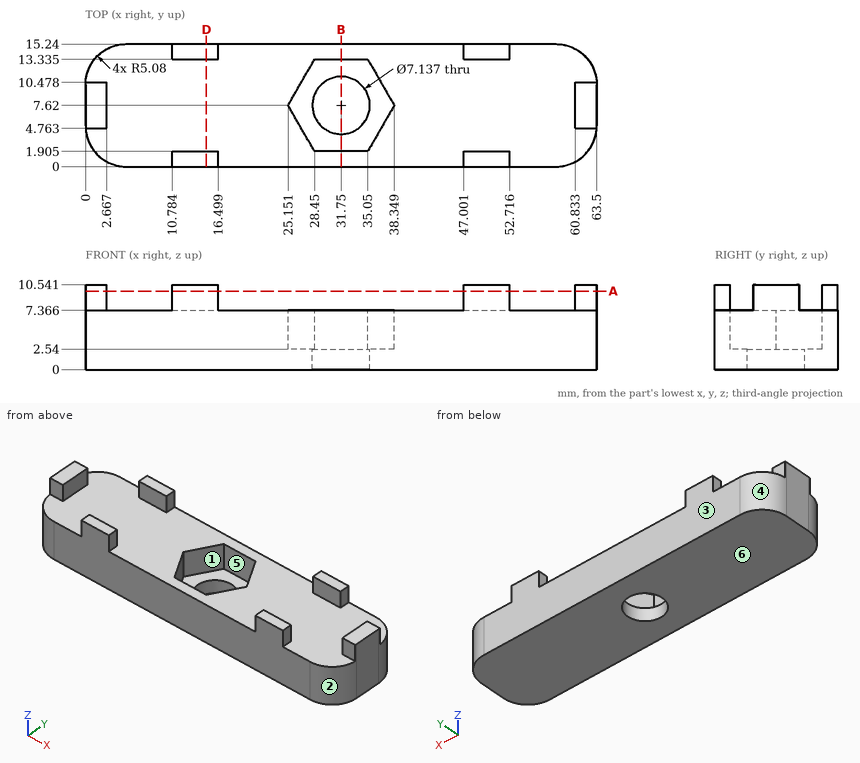
Verification items for this drawing (mm, ordinates from the low corner). A direction names the side the tool comes from. Coordinates: 2 decimals unless noted, no trailing zeros. Write each loop counter-clockwise with the first axis right and the second up, starting at its lowest first coordinate (ties: lowest second). Pieces come first, ordered by that corner, then holes. Notation, with made-up numbers: M 18.25,46.5 L 51.25,46.5 A22 cw 51.25,54.5 Z; hole C 36,4 d7. An arc over 180 degrees is marked long. Answer as a JSON object with one key per item and string values. Group by question number.
(1) Tool access check on the marked faces 5 and 6. Record the directions out of +Z, -Z, +X, -X, +Y, -Y that give a thin tool (end or side, any length) a straight path to the whole face; none if there is none.
(2) Cross-section at B-B, the plane x = 31.75. Record the cut outline in (y, z) (1 decimal).
(3) Gauge pin test, flat ends, axial feed: pin 1 (3 mm diameter, centred on x = 0.5, z = 9.5, fed in from -Y); pin 2 (0.6 mm diameter, centred on y = 14, z = 9, fed in from -X); pin 3 (1 mm diameter, centred on x = 51.5, y = 3, fed in from +Z). Record the tip position at first contact, or that the pin passes through.
(4) Cross-section at A-A, the plane z = 9.75. State how many separate pieces and enclosed holes the cut face has.
(5) Cross-section at D-D, the plane x = 15. Record the cut outline in (y, z) (1 decimal).
(6) Material ranges on line 1 (X direction, y = 14.5, z = 8.5) (1 decimal); line 2 (Y direction, x = 31.75, z = 1); line 3 (X direction, y = 6, z = 8.75), recorded low to high.
(7) Release check for a two-part mould opening along X. For the marked faces 1, 2, 3 and 4 record: +X half, -X half, draft (parallel to the pull), parting line (faces both ways), or undercut.
Reply:
{
 "1": {"face 5": "+Z", "face 6": "-Z, +X, -X, +Y, -Y"},
 "2": {"outline": "M 0,0 L 4.1,0 L 4.1,2.5 L 1.9,2.5 L 1.9,7.4 L 0,7.4 Z; M 11.2,0 L 15.2,0 L 15.2,7.4 L 13.3,7.4 L 13.3,2.5 L 11.2,2.5 Z"},
 "3": {"pin 1": "y = 4.76", "pin 2": "x = 10.78", "pin 3": "z = 7.37"},
 "4": {"separate pieces": "6", "enclosed holes": "0"},
 "5": {"outline": "M 0,0 L 15.2,0 L 15.2,10.5 L 13.3,10.5 L 13.3,7.4 L 1.9,7.4 L 1.9,10.5 L 0,10.5 Z"},
 "6": {"line 1": "10.8 to 16.5, 47 to 52.7", "line 2": "0 to 4.05, 11.19 to 15.24", "line 3": "0 to 2.67, 60.83 to 63.5"},
 "7": {"face 1": "undercut", "face 2": "+X half", "face 3": "draft", "face 4": "-X half"}
}
